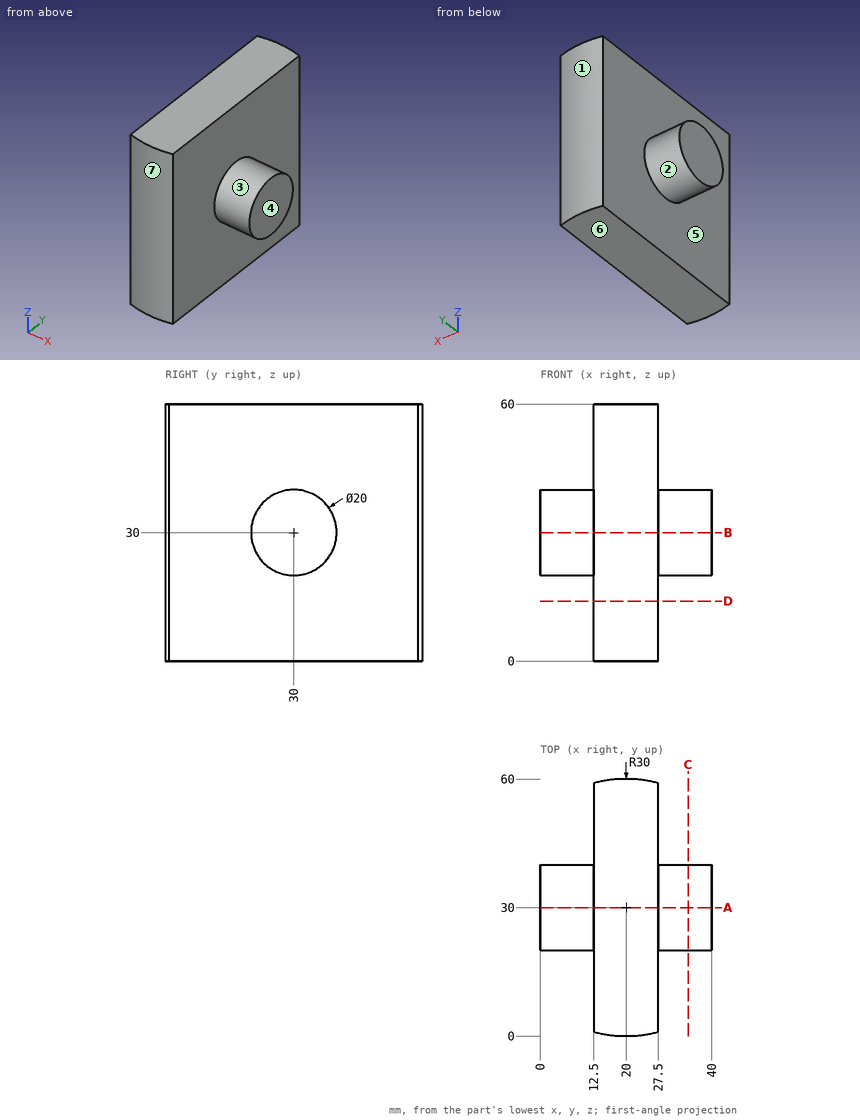
Answer from the drawing. Dimensions are ordinates in mm from the lowest x, y and z of the part. A direction names the side the tool comes from. Give positions to 0.01 mm unless a question says otherwise; leave off trailing zeros. Order: outer loops, then holes, each group sorted by start corner. A loop starts at its lowest first (then second) coordinate and runs counter-clockwise, first axis right, second up. Notation, with made-up numbers: (-7.75, 63) - (-3.75, 63) arc R32 cw to (-3.75, 100) - close; hole circle Ø7 at (48, -39.75). An arc over 180 degrees is marked (long way). One line per item, written item: value. Start each with the question number.
1) A tool of negligible diameter and unlimited length cuts with its end or side. For the marked faces 1, 2 and 3, from which of +Z, -Z, +X, -X, +Y, -Y can it reach the whole face along a straight path? Write none if from no direction.
2) The mould has two halves that part along X. Classify the marked faces 4, 5, 6 and 7: released by +X, released by -X, zero draft, split by the parting line, or undercut.
3) A cutting plane is placed at B-B on z = 30. Give the vertices of the cut face in (x, y), then the cut area to 3 significant figures.
4) A cutting plane is placed at D-D on z = 14. Give the vertices of the cut face in (x, y).
5) A cutting plane is placed at A-A on y = 30. Give the vertices of the cut face in (x, z), then the cut area to 3 significant figures.
6) Given pin 1 Ø10 at (x, z) = (12.5, 32.5) entering from -Y; pin 2 Ø2 at (y, z) = (49.5, 20.5) entering from +X; pin 3 Ø12 at (y, z) = (9.5, 51.5) entering from -X; pin 4 Ø17.5 at (y, z) = (33.5, 17.5) entering from +X, each flat-ended and moving along its own axis, determine where each tip first touches the part or whether it passes through.
7) Find the intervals of material crossed by L1, parallel to X at y = 50.5, z = 30.5; L2, parallel to Y at x = 20, z = 49.5; L3, parallel to Y at x = 30, z = 30.5, in increasing order.
8) A cutting plane is placed at C-C on x = 34.5. Give the vertices of the cut face in (y, z).
Answer sheet:
1. face 1: +Z, -Z, +Y
1. face 2: -X
1. face 3: +X
2. face 4: released by +X
2. face 5: released by -X
2. face 6: zero draft
2. face 7: split by the parting line
3. outline: (0, 20) - (12.5, 20) - (12.5, 0.95) arc R30 ccw to (27.5, 0.95) - (27.5, 20) - (40, 20) - (40, 40) - (27.5, 40) - (27.5, 59.05) arc R30 ccw to (12.5, 59.05) - (12.5, 40) - (0, 40) - close
3. area: 1,390 mm2
4. outline: (12.5, 0.95) arc R30 ccw to (27.5, 0.95) - (27.5, 59.05) arc R30 ccw to (12.5, 59.05) - close
5. outline: (0, 20) - (12.5, 20) - (12.5, 0) - (27.5, 0) - (27.5, 20) - (40, 20) - (40, 40) - (27.5, 40) - (27.5, 60) - (12.5, 60) - (12.5, 40) - (0, 40) - close
5. area: 1,400 mm2
6. pin 1: stops at y = 0.1
6. pin 2: stops at x = 27.5
6. pin 3: stops at x = 12.5
6. pin 4: stops at x = 40
7. L1: x = 12.5 to 27.5
7. L2: y = 0 to 60
7. L3: y = 20.01 to 39.99
8. outline: circle Ø20 at (30, 30)
